Can you work these out from the model? Positions are in its coordinate system, mm. A direction names the side the tool comes from. Coordinates: 2 decimals unless noted, no trailing zeros. Loops run counter-clockwise (first coordinate to the right, second up) from the corner with the lowest first, then second, coordinate; pieces in that order, holes last. Notation, with made-up numbers: M -21.75,-34.5 L 5.25,-34.5 A26 cw 5.25,3.5 Z; hole C -19,-7.5 d7. An arc over 180 degrees is marked long. Answer as a JSON object with one key per item and string values. Group by question number.
Item 1: Which directions (+Z, -Z, +X, -X, +Y, -Y) give clear straight access to the entire face, cutting with the end or side of a thin tool? Please do faces 1 (the flat face through (19, -19, 78)), 2 (the flat face through (-19, 19, 78)), 3 (the flat face through (-19, -19, 78)).
Item 2: Suppose I cut it at D-D (z = 67). Write out the boundary of the cut face in (x, y).
Item 3: If I drill on line 1 (Y direction, x = 19, z = 9.5); line 2 (Z direction, x = 17.5, y = -21.5); line 3 (X direction, y = -18.5, z = 17.5), over which ranges is the centre line in solid material (lowest first)?
Item 4: Suppose I cut it at C-C (z = 24). Write out the boundary of the cut face in (x, y), then the cut area to 3 significant figures.
Item 5: Suppose I cut it at B-B (x = 28.5). Write out the boundary of the cut face in (y, z).
Item 6: Suppose I cut it at A-A (y = 27). Write out the boundary of the cut face in (x, z), then the cut area to 3 significant figures.
Item 7: I'm going to push flat-ended pins straight in: pin 1 Ø12 at (x, z) = (-30, 13) entering from +Y; pin 2 Ø4 at (y, z) = (-25.5, 53.5) entering from -X. Where does each tip first touch, or does it pass through?
```python
from build123d import *

# Parameters (mm, degrees)
F0_W     = 38
F0_H     = 38
F1_DEPTH = 76
F5_COUNT = 4
F8_DEPTH = 5


with BuildPart() as f1:
    # F0 (on Top) → F1 (new body)
    with BuildSketch(Plane.XY):
        with Locations((-19, 19)):
            Rectangle(F0_W, F0_H)
    extrude(amount=F1_DEPTH)

    # F4: sweep along a path in F2
    with BuildLine(Plane.XY) as f4_path:
        Line((-76, -38), (0, 38))
    # F3 (on face) → F4 (sweep, cut)
    with BuildSketch(Plane(origin=(-38, 0, 0), x_dir=(0, -1, 0), z_dir=(-1, 0, 0))):
        Polygon((-38, 76), (-38, 38), (0, 76), align=None)
        Polygon((-38, 0), (0, 0), (-38, 38), align=None)
    sweep(path=f4_path.line, mode=Mode.SUBTRACT)


with BuildPart() as f5_1:
    # F5: instance of F1
    add(f1.part.rotate(Axis((0, 0, 38), (0, 0, 1)), 1 * 360 / F5_COUNT))


with BuildPart() as f5_2:
    # F5: instance of F1
    add(f1.part.rotate(Axis((0, 0, 38), (0, 0, 1)), 2 * 360 / F5_COUNT))


with BuildPart() as f5_3:
    # F5: instance of F1
    add(f1.part.rotate(Axis((0, 0, 38), (0, 0, 1)), 3 * 360 / F5_COUNT))


with BuildPart() as f5_1_1:
    add(f5_1.part)

    # F6: union F1, F5_3, F5_2
    add(f1.part)
    add(f5_3.part)
    add(f5_2.part)

    # F7 (on face) → F8 (join)
    with BuildSketch(Plane.XY.offset(76)):
        Polygon((-38, 0), (0, -38), (38, 0), (0, 38), align=None)
    extrude(amount=F8_DEPTH)


solid = f5_1_1.part
```
From the geometry:
{
 "1": {"face 1": "+Z, +X, -Y", "face 2": "+Z, -X, +Y", "face 3": "+Z, -X, -Y"},
 "2": {"outline": "M -38,-9 L -9,-38 L 9,-38 L 38,-9 L 38,9 L 9,38 L -9,38 L -38,9 Z"},
 "3": {"line 1": "-28.5 to 28.5", "line 2": "1 to 75", "line 3": "-37 to 37"},
 "4": {"outline": "M -38,-24 L -24,-38 L 24,-38 L 38,-24 L 38,24 L 24,38 L -24,38 L -38,24 Z", "area": "5,380 mm2"},
 "5": {"outline": "M -38,28.5 L -9.5,0 L 9.5,0 L 38,28.5 L 38,47.5 L 9.5,76 L 9.5,81 L -9.5,81 L -9.5,76 L -38,47.5 Z"},
 "6": {"outline": "M -38,27 L -11,0 L 11,0 L 38,27 L 38,49 L 11,76 L 11,81 L -11,81 L -11,76 L -38,49 Z", "area": "4,430 mm2"},
 "7": {"pin 1": "y = 29.49", "pin 2": "x = -37.83"}
}
